Check sheet for the modelled part. Datum: model origin and axes. Units: mm. Face numbers are marked on the shaded views. Round coordinates to 2 decimals unless told otherwise and drop trailing zeros. Write each loop counter-clockwise with the first axis right and the second up, starting at its lowest first coordinate (ties: lowest second). Pieces come first, ordered by that corner, then holes. Notation, with made-up numbers: (20.25, 11.25) -> (60.25, 11.25) arc R25 cw to (60.25, 39.25) -> close; hole circle Ø1 at (-34, 86.25). An arc over 180 degrees is marked (long way). One line per item, written item: value.
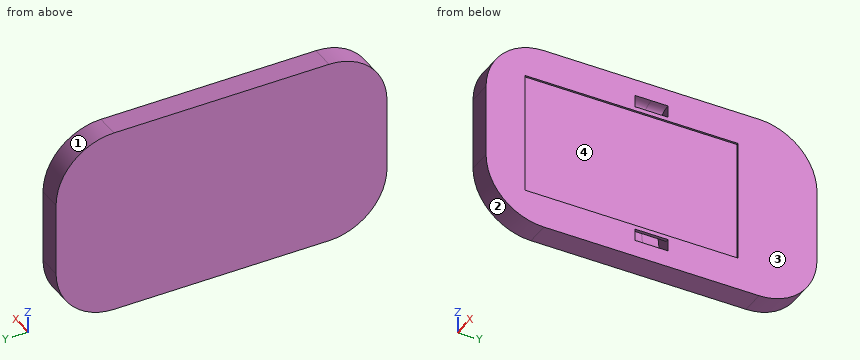
Autodesk Inventor part; units mm, degrees
ref_plane "YZ Plane" through (0, 0, 0) normal (1, 0, 0) x (0, 1, 0)
ref_plane "XZ Plane" through (0, 0, 0) normal (0, 1, 0) x (-1, 0, 0)
ref_plane "XY Plane" through (0, 0, 0) normal (0, 0, 1) x (1, 0, 0)
ref_plane "Work Plane2" through (0, 0, 0) normal (1, 0, 0) x (0, 0, -1)
sketch "Sketch1" plane through (0, 0, 0) normal (1, 0, 0) x (0, 0, -1)
  line L0 (20, -35) -> (-20, -35)
  line L1 (-20, -35) -> (-20, 35)
  line L2 (-20, 35) -> (20, 35)
  line L3 (20, 35) -> (20, -35)
  line L4 (20, -35) -> (-20, 35) construction
  line L5 (-20, -35) -> (20, 35) construction
  point P0 (0, 0)
  dimension "d0" = 40
  dimension "d1" = 70
extrude "Extrusion1" add sketch "Sketch1" along normal blind 5
fillet "Fillet1" radius 12.25 4 edges at (2.5, -35, 20) (2.5, -35, -20) (2.5, 35, -20) (2.5, 35, 20)
sketch "Sketch2" plane through (0, 0, 0) normal (-1, 0, 0) x (0, 0, 1)
  circle A0 centre (0, -20.5) radius 6.6
  line L0 (30.2912, 0) -> (32.4021, 0)
  circle A1 centre (0, 20.5) radius 6.6
  point P0 (0, 0)
  dimension "d5" = 13.2
  dimension "d17" = 41
extrude "Extrusion2" cut sketch "Sketch2" against normal blind 3.75
sketch "Sketch3" plane through (0, 0, 0) normal (-1, 0, 0) x (0, 0, 1)
  circle A0 centre (0, 20.5) radius 6.6
  circle A1 centre (0, -20.5) radius 6.6
  point P0 (0, 0)
extrude "Extrusion3" add sketch "Sketch3" against normal blind 0.4
sketch "Sketch4" plane through (5, 0, 0) normal (1, 0, 0) x (0, 0, -1)
  line L0 (13, -26.7517) -> (-13, -26.7517)
  line L1 (-13, -26.7517) -> (-13, 18.2483)
  line L2 (-13, 18.2483) -> (13, 18.2483)
  line L3 (13, 18.2483) -> (13, -26.7517)
  line L4 (13, -26.7517) -> (-13, 18.2483) construction
  line L5 (-13, -26.7517) -> (13, 18.2483) construction
  point P0 (0, -4.2517)
  point P1 (0, 0)
  dimension "d10" = 26
  dimension "d11" = 45
  dimension "d12" = 0
extrude "Extrusion4" cut sketch "Sketch4" against normal blind 0.4
sketch "Sketch6" plane through (0, 0, 0) normal (0, 1, 0) x (-1, 0, 0)
  line L0 (5.3087, 0) -> (6.8591, 0)
  line L1 (-5, -20) -> (-5, -7.75)
  line L2 (-5, -13.875) -> (-3.2306, -14.0634) construction
  line L3 (-3.2306, -14.0634) -> (-2.8267, -12.0185) construction
  line L4 (-2.8267, -12.0185) -> (-2.8267, -8.1465) construction
  line L5 (-2.8267, -8.1465) -> (-2.8267, 0) construction
  spline S0 degree 4 poles (-5, -13.875) (-3.2306, -14.0634) (-2.8267, -12.0185) (-2.8267, -8.1465) (-2.8267, 0) knots 1 1 1 1 1 2 2 2 2 2
  line L6 (-5, -16.4324) -> (-0.7919, -16.4324) construction
  line L7 (-0.7919, -16.4324) -> (-0.9641, -12.8693) construction
  line L8 (-0.9641, -12.8693) -> (-0.7919, -3.5174) construction
  line L9 (-0.7919, -3.5174) -> (-0.7919, 0) construction
  line L10 (-0.4, -6.6) -> (-3.75, -6.6)
  spline S1 degree 4 poles (-5, -16.4324) (-0.7919, -16.4324) (-0.9641, -12.8693) (-0.7919, -3.5174) (-0.7919, 0) knots 1 1 1 1 1 2 2 2 2 2
  line L11 (-5, -16.4324) -> (-5, -13.875)
  line L12 (-2.8267, 0) -> (-0.7919, 0)
  line L13 (-5, 13.875) -> (-3.2306, 14.0634) construction
  line L14 (-3.2306, 14.0634) -> (-2.8267, 12.0185) construction
  line L15 (-2.8267, 12.0185) -> (-2.8267, 8.1465) construction
  line L16 (-2.8267, 8.1465) -> (-2.8267, 0) construction
  spline S2 degree 4 poles (-5, 13.875) (-3.2306, 14.0634) (-2.8267, 12.0185) (-2.8267, 8.1465) (-2.8267, 0) knots 1 1 1 1 1 2 2 2 2 2
  line L17 (-5, 16.4324) -> (-0.7919, 16.4324) construction
  line L18 (-0.7919, 16.4324) -> (-0.9641, 12.8693) construction
  line L19 (-0.9641, 12.8693) -> (-0.7919, 3.5174) construction
  line L20 (-0.7919, 3.5174) -> (-0.7919, 0) construction
  spline S3 degree 4 poles (-5, 16.4324) (-0.7919, 16.4324) (-0.9641, 12.8693) (-0.7919, 3.5174) (-0.7919, 0) knots 1 1 1 1 1 2 2 2 2 2
  line L21 (-5, -13.875) -> (-5, -16.4324)
  line L22 (-5, 13.875) -> (-5, 16.4324)
  point P0 (0, 0)
extrude "Extrusion5" cut sketch "Sketch6" along normal mid plane 7
properties part number "Sentroller_Mount"
Item 1: Depth check by flat-ended pin: P1, Ø1, axis at x = 3.5, z = 15.5, coming from the -Y side; P2, Ø8, axis at y = -20.5, z = 0, coming from the +X side. Enter the tip coordinate at first touch or a pass-through.
Answer:
P1: stops at y = -32.62
P2: stops at x = 4.6
Item 2: Sectioned sample at B-B on y = 4.5. Enter the section's corners in (x, z).
Answer:
outline: (0, -20) -> (5, -20) -> (5, -13) -> (4.6, -13) -> (4.6, 13) -> (5, 13) -> (5, 20) -> (0, 20) -> close
Item 3: Sectioned sample at D-D on y = -20.5. Enter the section's corners in (x, z), and give its area (3 significant figures).
Answer:
outline: (0, -20) -> (5, -20) -> (5, -13) -> (4.6, -13) -> (4.6, 13) -> (5, 13) -> (5, 20) -> (0, 20) -> close; hole (0.4, -6.6) -> (3.75, -6.6) -> (3.75, 6.6) -> (0.4, 6.6) -> close
area: 145 mm^2
Item 4: Thickness scan on line 1 (Y direction, x = 2.6, z = 0); line 2 (Y direction, x = 2.9, z = 0); line 3 (X direction, y = 24, z = 5). Record the ranges inside material, lowest first.
Answer:
line 1: y = -35 to -27.1, -13.9 to -3.5, 3.5 to 13.9, 27.1 to 35
line 2: y = -35 to -27.1, -13.9 to 13.9, 27.1 to 35
line 3: x = 0 to 0.4, 3.75 to 5
Item 5: Mould release check, pull along Y, two halves, no side actions. Record for the marked faces 1, 2, 3 and 4: pulls with the +Y half, pulls with the -Y half, needs draft (parallel to the pull), parting line crosses it, or undercut.
Answer:
face 1: pulls with the +Y half
face 2: pulls with the -Y half
face 3: needs draft
face 4: undercut
Item 6: Sectioned sample at C-C on x = 1.55. Count the separate pieces of the cut face and the enclosed holes in it, and give its area (3 significant figures).
Answer:
separate pieces: 1
enclosed holes: 3
area: 2,210 mm^2
Item 7: Sectioned sample at A-A on y = 20.5. Enter the section's corners in (x, z), and give its area (3 significant figures).
Answer:
outline: (0, -20) -> (5, -20) -> (5, 20) -> (0, 20) -> close; hole (0.4, -6.6) -> (3.75, -6.6) -> (3.75, 6.6) -> (0.4, 6.6) -> close
area: 156 mm^2
